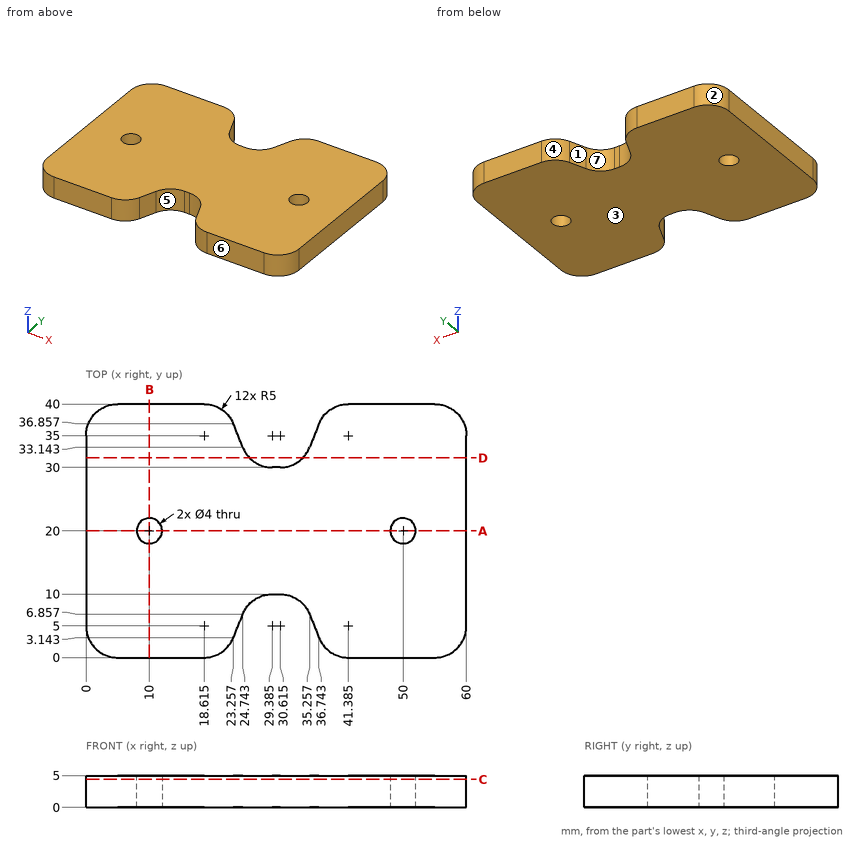
Could you check a few things on this drawing? It's one solid part, dimensions in mm from its lowest x, y, z. A direction names the side the tool comes from. Coordinates: 2 decimals unless noted, no trailing zeros. Order: outer loops, then holes, each group sorted by start corner. A loop starts at its lowest first (then second) coordinate and runs counter-clockwise, first axis right, second up. Notation, with made-up numbers: M 81,-19.5 L 100,-19.5 A28 cw 100,7.5 Z; hole C 80,-3.75 d9. An arc over 180 degrees is marked long. Use one line per item in the form item = value. Start each with the question number.
1. Suppose I cut it at A-A on y = 20. Write out the boundary of the cut face in (x, z).
2. For pin 1 (2.5 mm diameter, centred on x = 50, y = 20, fed in from +Z); pin 2 (1 mm diameter, centred on x = 30, z = 2.5, fed in from +Y); pin 3 (1 mm diameter, centred on x = 21.5, z = 4, fed in from -Y) (1 decimal), each with a flat end and sliding along its axis, tell me the tip position at first contact or that it passes through.
3. On a 3-axis mill with a long thin cutter (end or side, diameter ignored), from which of +Z, -Z, +X, -X, +Y, -Y can I reach the whole of each face in a straight line? I mean the marked faces 5, 6 and 7. Say none if no direction works.
4. We'd pull the mould along X, two halves only. Please class the marked faces 1, 2, 3 and 4: +X half, -X half, draft (parallel to the pull), parting line (faces both ways), or undercut.
5. Suppose I cut it at B-B on x = 10. Write out the boundary of the cut face in (y, z), then the cut area to 3 significant figures.
6. Suppose I cut it at D-D on y = 31.5. Write out the boundary of the cut face in (x, z).
7. Please list where these lines run through material, in increasing order: line 1 (Y direction, x = 50, z = 3.1); line 2 (X direction, y = 21, z = 3.1); line 3 (X direction, y = 18.5, z = 4.4).
8. Suppose I cut it at C-C on z = 4.4. Write out the boundary of the cut face in (x, y) (1 decimal), then the cut area to 3 significant figures.
Geometry says:
q1.outline = M 0,0 L 8,0 L 8,5 L 0,5 Z; M 12,0 L 48,0 L 48,5 L 12,5 Z; M 52,0 L 60,0 L 60,5 L 52,5 Z
q2.pin_1 = through
q2.pin_2 = 30
q2.pin_3 = 0.6
q3.face_5 = +Z, -Z, -Y
q3.face_6 = +Z, -Z, +X, -X, -Y
q3.face_7 = +Z, -Z, +Y
q4.face_1 = undercut
q4.face_2 = -X half
q4.face_3 = draft
q4.face_4 = undercut
q5.outline = M 0,0 L 18,0 L 18,5 L 0,5 Z; M 22,0 L 40,0 L 40,5 L 22,5 Z
q5.area = 180 mm^2
q6.outline = M 0,0 L 25.81,0 L 25.81,5 L 0,5 Z; M 34.19,0 L 60,0 L 60,5 L 34.19,5 Z
q7.line_1 = 0 to 18, 22 to 40
q7.line_2 = 0 to 8.27, 11.73 to 48.27, 51.73 to 60
q7.line_3 = 0 to 8.68, 11.32 to 48.68, 51.32 to 60
q8.outline = M 0,5 A5 ccw 5,0 L 18.6,0 A5 ccw 23.3,3.1 L 24.7,6.9 A5 cw 29.4,10 L 30.6,10 A5 cw 35.3,6.9 L 36.7,3.1 A5 ccw 41.4,0 L 55,0 A5 ccw 60,5 L 60,35 A5 ccw 55,40 L 41.4,40 A5 ccw 36.7,36.9 L 35.3,33.1 A5 cw 30.6,30 L 29.4,30 A5 cw 24.7,33.1 L 23.3,36.9 A5 ccw 18.6,40 L 5,40 A5 ccw 0,35 Z; hole C 10,20 d4; hole C 50,20 d4
q8.area = 2,110 mm^2
